Design review of the part shown in the three views and the two pictorial views. Dimensions are in mm from the part's minimum x, y and z. Give positions to 0.01 mm unless a question says otherwise; leave off trailing zeros. Loops run counter-clockwise (first coordinate to the right, second up) from the corner with the lowest first, then second, coordinate; pieces in that order, holes last. Notation, with made-up numbers: (48, -9) - (74, -9) arc R10 cw to (74, 3) - close; hole circle Ø8 at (44.25, -17.5). An arc over 180 degrees is marked (long way). Return JSON: item names as keys, results as strings. Group by question number.
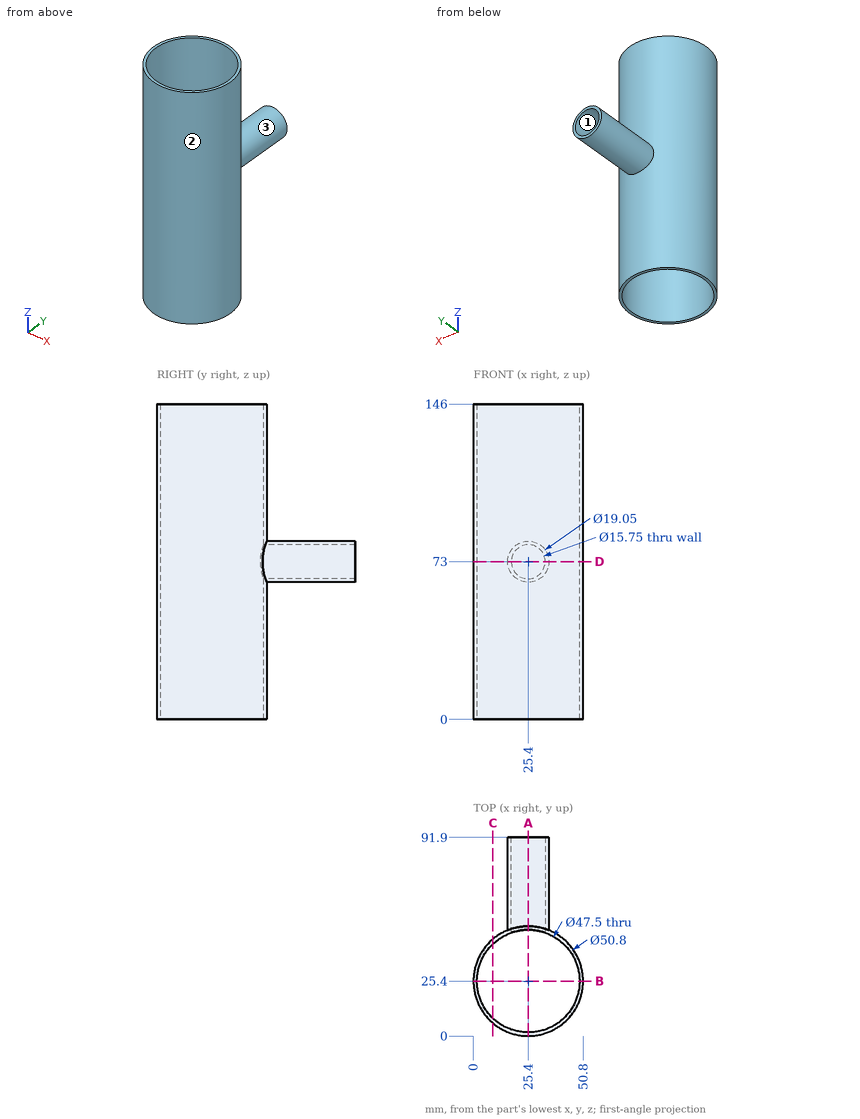
Item 1: For L1, parallel to Z at x = 25, y = 63; L2, parallel to Y at x = 25.4, z = 48.5; L3, parallel to Y at x = 23, z = 120, list the stretches that pass through material, from the lowest coordinate up. Write a range as from..to.
Item 2: For P1, Ø8, axis at x = 14.5, y = 58.5, coming from the -Z side; P2, Ø2, axis at y = 34, z = 111.5, coming from the -X side; P3, Ø1, axis at x = 14.5, z = 49, coming from the -Y side, all flat-tipped, find the tip position at first contact; note any pin that passes through.
Item 3: Take a section at B-B (y = 25.4). State the section outline as (x, z) points, then the cut area to 3 significant figures.
Item 4: Take a section at A-A (x = 25.4). State the section outline as (y, z) points (3 decimals), then the cut area to 3 significant figures.
Item 5: Mouldability with a two-part tool opening along Z and no side actions: class the marked faces 1, 2 and 3 as +Z half, -Z half, draft (parallel to the pull), parting line (faces both ways), or undercut.
Item 6: Take a section at C-C (x = 9). State the section outline as (y, z) points.
Item 7: Take a section at D-D (z = 73). State the section outline as (x, y) points (3 decimals), then the cut area to 3 significant figures.
Check sheet entries:
{
 "1": {"L1": "z = 63.48..65.14, 80.86..82.52", "L2": "y = 0..1.65, 49.15..50.8", "L3": "y = 0.11..1.77, 49.03..50.69"},
 "2": {"P1": "stops at z = 66.43", "P2": "stops at x = 1.16", "P3": "stops at y = 2.23"},
 "3": {"outline": "(0, 0) - (1.65, 0) - (1.65, 146) - (0, 146) - close; (49.15, 0) - (50.8, 0) - (50.8, 146) - (49.15, 146) - close", "area": "482 mm^2"},
 "4": {"outline": "(0, 0) - (1.65, 0) - (1.65, 146) - (0, 146) - close; (49.15, 0) - (50.8, 0) - (50.8, 63.475) - (91.9, 63.475) - (91.9, 65.125) - (49.15, 65.125) - close; (49.15, 80.875) - (91.9, 80.875) - (91.9, 82.525) - (50.8, 82.525) - (50.8, 146) - (49.15, 146) - close", "area": "591 mm^2"},
 "5": {"face 1": "undercut", "face 2": "draft", "face 3": "parting line"},
 "6": {"outline": "(6, 0) - (8.22, 0) - (8.22, 146) - (6, 146) - close; (42.58, 0) - (44.8, 0) - (44.8, 146) - (42.58, 146) - close"},
 "7": {"outline": "(15.875, 48.946) arc R25.4 ccw (long way) to (34.925, 48.946) - (34.925, 91.9) - (33.275, 91.9) - (33.275, 47.806) arc R23.75 cw (long way) to (17.525, 47.806) - (17.525, 91.9) - (15.875, 91.9) - close", "area": "369 mm^2"}
}
